Job drawing, mm, ordinate dimensions from the low corner. One solid piece. Coordinates: 2 decimals unless noted, no trailing zeros. Loops run counter-clockwise (first coordinate to the right, second up) from the corner with the lowest first, then second, coordinate; pieces in that order, holes last. Notation, with made-up numbers: (83, 85.5) -> (107, 85.5) arc R15 cw to (107, 105.5) -> close; hole circle Ø10 at (63.5, 0.25). An arc over 180 degrees is marked (long way). Answer as CSV lines item,"result". Start each with the question number.
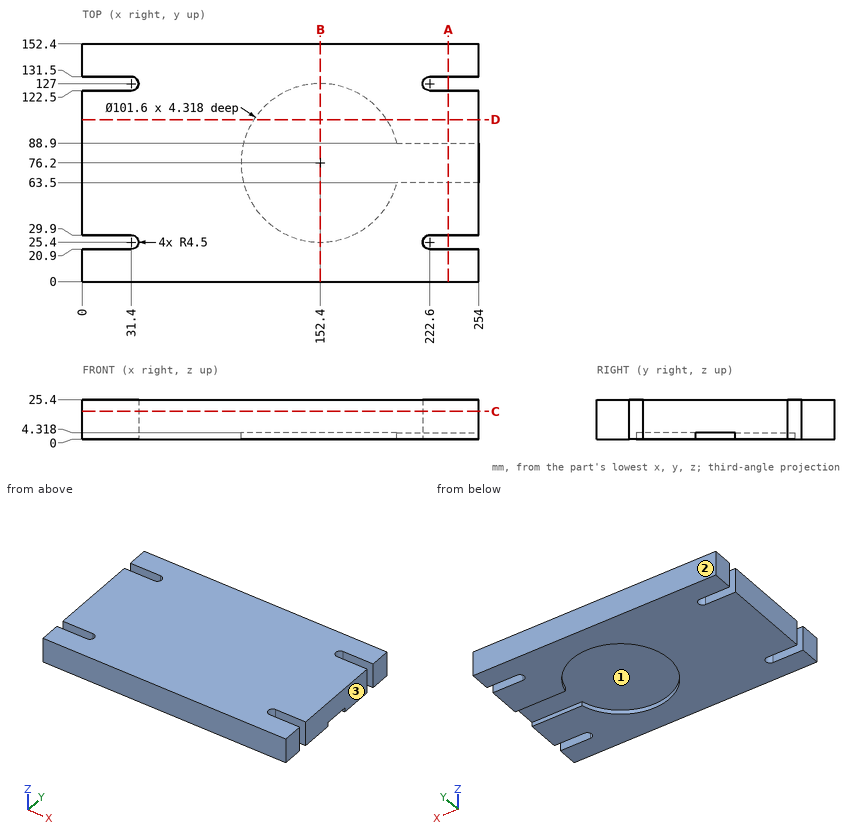
Q1. Saw through at D-D (y = 104). List the corners of the cut face in (x, z).
Q2. Probe probe 1 along Y at (x, z) = (242.5, 12); probe 2 along Y at (x, z) = (152.4, 1.8); probe 3 along Z at (x, y) = (209, 64.5). List the from-to ranges inside material, lowest first. Write a range as from..to.
Q3. Saw through at B-B (x = 152.4). List the corners of the cut face in (y, z).
Q4. Saw through at A-A (x = 234.5). List the corners of the cut face in (y, z).
Q5. Pin check, flat tip, straight feed: pin 1 Ø4 at (x, z) = (215, 8.5) entering from -Y. Stop position of the tip, or through.
Q6. Two-plate mould, pull along X, no slides. Class the marked faces 1, 2 and 3: pulls with the +X half, pulls with the -X half, needs draft (parallel to the pull), parting line crosses it, or undercut.
Q7. Saw through at C-C (z = 18). List the corners of the cut face in (x, y), and give its area (3 significant figures).
Ans:
1,outline,"(0, 0) -> (109.88, 0) -> (109.88, 4.32) -> (194.92, 4.32) -> (194.92, 0) -> (254, 0) -> (254, 25.4) -> (0, 25.4) -> close"
2,probe 1,"y = 0..20.9, 29.9..122.5, 131.5..152.4"
2,probe 2,"y = 0..25.4, 127..152.4"
2,probe 3,"z = 4.32..25.4"
3,outline,"(0, 0) -> (25.4, 0) -> (25.4, 4.32) -> (127, 4.32) -> (127, 0) -> (152.4, 0) -> (152.4, 25.4) -> (0, 25.4) -> close"
4,outline,"(0, 0) -> (20.9, 0) -> (20.9, 25.4) -> (0, 25.4) -> close; (29.9, 0) -> (63.5, 0) -> (63.5, 4.32) -> (88.9, 4.32) -> (88.9, 0) -> (122.5, 0) -> (122.5, 25.4) -> (29.9, 25.4) -> close; (131.5, 0) -> (152.4, 0) -> (152.4, 25.4) -> (131.5, 25.4) -> close"
5,pin 1,"stops at y = 0"
6,face 1,"undercut"
6,face 2,"needs draft"
6,face 3,"pulls with the +X half"
7,outline,"(0, 0) -> (254, 0) -> (254, 20.9) -> (222.6, 20.9) arc R4.5 cw to (222.6, 29.9) -> (254, 29.9) -> (254, 122.5) -> (222.6, 122.5) arc R4.5 cw to (222.6, 131.5) -> (254, 131.5) -> (254, 152.4) -> (0, 152.4) -> (0, 131.5) -> (31.4, 131.5) arc R4.5 cw to (31.4, 122.5) -> (0, 122.5) -> (0, 29.9) -> (31.4, 29.9) arc R4.5 cw to (31.4, 20.9) -> (0, 20.9) -> close"
7,area,"37,500 mm²"
